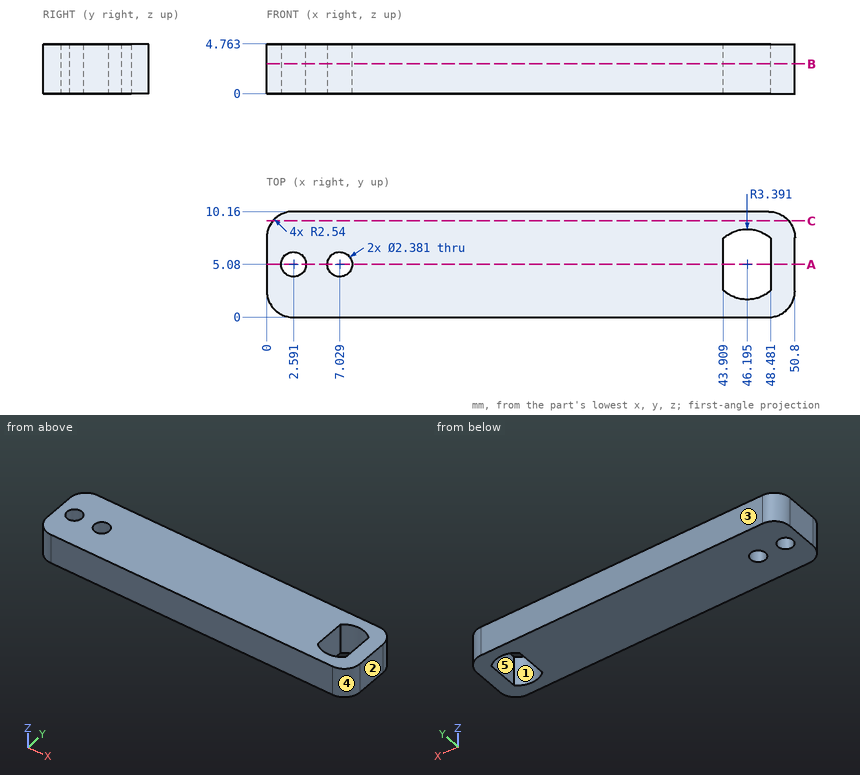
For this review, use the dimensioned drawing (mm, ordinates from the lowest corner) and the shaded views. A direction names the side the tool comes from. Round coordinates to 2 decimals unless told otherwise and drop trailing zeros. Order: outer loops, then holes, each group sorted by start corner. A loop starts at its lowest first (then second) coordinate and runs counter-clockwise, first axis right, second up.
1) Consider section A-A (y = 5.08). State the section outline as (x, z) points.
The answers:
outline: (0, 0) - (1.4, 0) - (1.4, 4.76) - (0, 4.76) - close; (3.78, 0) - (5.84, 0) - (5.84, 4.76) - (3.78, 4.76) - close; (8.22, 0) - (43.91, 0) - (43.91, 4.76) - (8.22, 4.76) - close; (48.48, 0) - (50.8, 0) - (50.8, 4.76) - (48.48, 4.76) - close
2) For L1, parallel to X at y = 5, z = 0.55; L2, parallel to X at y = 4.5, z = 3.75; L3, parallel to Y at x = 7, z = 2.1, list the stretches that pass through material, from the lowest coordinate up.
The answers:
L1: x = 0 to 1.4, 3.78 to 5.84, 8.22 to 43.91, 48.48 to 50.8
L2: x = 0 to 1.55, 3.63 to 5.99, 8.07 to 43.91, 48.48 to 50.8
L3: y = 0 to 3.89, 6.27 to 10.16
3) Consider section C-C (y = 9.25). State the section outline as (x, z) points.
The answers:
outline: (0.59, 0) - (50.21, 0) - (50.21, 4.76) - (0.59, 4.76) - close
4) Machinability: for the marked faces 4 and 5, which of the approach directions +Z, -Z, +X, -X, +Y, -Y give a long, thin tool a straight path to every point of the face, cutting with its end or side? Answer none if there is none.
The answers:
face 4: +Z, -Z, +X, -Y
face 5: +Z, -Z
5) Draft analysis for pull direction X (two halves, no side actions). For the marked faces 1, 2 and 3, state which applies: released by +X, released by -X, zero draft, split by the parting line, or undercut.
The answers:
face 1: undercut
face 2: released by +X
face 3: zero draft
6) Consider section B-B (z = 2.85). State the section outline as (x, y) points (1 decimal), plus the area to 3 significant figures.
The answers:
outline: (0, 2.5) arc R2.5 ccw to (2.5, 0) - (48.3, 0) arc R2.5 ccw to (50.8, 2.5) - (50.8, 7.6) arc R2.5 ccw to (48.3, 10.2) - (2.5, 10.2) arc R2.5 ccw to (0, 7.6) - close; hole circle Ø2.4 at (2.6, 5.1); hole circle Ø2.4 at (7, 5.1); hole (43.9, 2.6) arc R3.4 ccw to (48.5, 2.6) - (48.5, 7.6) arc R3.4 ccw to (43.9, 7.6) - close
area: 473 mm2
